Autodesk Inventor part; units mm, degrees
ref_plane "YZ Plane" through (0, 0, 0) normal (1, 0, 0) x (0, 1, 0)
ref_plane "XZ Plane" through (0, 0, 0) normal (0, 1, 0) x (-1, 0, 0)
ref_plane "XY Plane" through (0, 0, 0) normal (0, 0, 1) x (1, 0, 0)
sketch "Skizze1" plane through (0, 0, 0) normal (0, 0, 1) x (1, 0, 0)
  line L0 (-70, 25) -> (-70, 40)
  line L1 (-70, 40) -> (-80, 40)
  line L2 (-80, 40) -> (-80, 0)
  line L3 (-80, 0) -> (77, 0)
  line L4 (77, 0) -> (77, 25)
  line L5 (72, 25) -> (72, 23)
  line L6 (72, 23) -> (70, 23)
  line L7 (70, 23) -> (70, 25)
  line L8 (77, 25) -> (72, 25)
  line L9 (70, 25) -> (-70, 25)
  dimension "d0" = 80
  dimension "d1" = 10
  dimension "d2" = 50
  dimension "d3" = 46
  dimension "d7" = 2
  dimension "d8" = 5
  dimension "d13" = 140
revolve "Drehung1" add sketch "Skizze1" angle 360 about axis through (-80, 0, 0) along (1, 0, 0)
chamfer "Fase1" distance 2 angle 45 1 edges at (-80, -40, 0)
chamfer "Fase2" distance 2 angle 45 1 edges at (77, -25, 0)
properties part number "Boltx50"
Here's how the part is built. I have some questions about the finished solid (model axes, mm). A direction names the side the tool comes from. Give positions to 0.01 mm unless a question says otherwise; leave off trailing zeros. Order: outer loops, then holes, each group sorted by start corner. A loop starts at its lowest first (then second) coordinate and runs counter-clockwise, first axis right, second up. Notation, with made-up numbers: M -13.5,-6 L 7.5,-6 A17 ccw 7.5,0 Z; hole C -15.75,4.25 d3. An arc over 180 degrees is marked long. Answer as a JSON object with one key per item and string values. Group by question number.
1) I'm going to push flat-ended pins straight in: pin 1 Ø6 at (x, y) = (-52, -14.5) entering from +Z; pin 2 Ø2 at (x, y) = (-3, -5.5) entering from -Z; pin 3 Ø8 at (x, y) = (-42, -3.5) entering from +Z. Where does each tip first touch, or does it pass through?
2) On a 3-axis mill with a long thin cutter (end or side, diameter ignored), from which of +Z, -Z, +X, -X, +Y, -Y can I reach the whole of each face in a straight line? I mean faces 1 (the flat face through (-70, 17.22, 18.34)), 2 (the flat face through (77, 0, 0)), 3 (the flat face through (70, 22.1, -7.3)). Say none if no direction works.
3) We'd pull the mould along X, two halves only. Please class faces 4 (the flat face through (72, 22.1, -7.3)), 5 (the conical face through (-79.875, -4.963, 37.801)), 6 (the cylindrical face through (-74.06, -8.67, 39.05)): pulls with the +X half, pulls with the -X half, needs draft (parallel to the pull), parting line crosses it, or undercut.
4) Suppose I cut it at C-C, the plane x = 38. Write out the boundary of the cut face in (y, z), plus the area to 3 significant figures.
5) Please list where these lines run through material, in increasing order: L1, parallel to X at y = -24.5, z = -29; L2, parallel to Y at x = 21, z = -4.5; L3, parallel to Y at x = -34, z = -6. Write a range as [from, to].
6) Suppose I cut it at A-A, the plane y = 0. Write out the boundary of the cut face in (x, z).
Results found:
{
 "1": {"pin 1": "z = 22.2", "pin 2": "z = -24.59", "pin 3": "z = 25"},
 "2": {"face 1": "+X", "face 2": "+Z, -Z, +X, +Y, -Y", "face 3": "none"},
 "3": {"face 4": "undercut", "face 5": "pulls with the -X half", "face 6": "needs draft"},
 "4": {"outline": "C 0,0 d50", "area": "1,960 mm²"},
 "5": {"L1": "[-80, -70]", "L2": "[-24.59, 24.59]", "L3": "[-24.27, 24.27]"},
 "6": {"outline": "M -80,-38 L -78,-40 L -70,-40 L -70,-25 L 70,-25 L 70,-23 L 72,-23 L 72,-25 L 75,-25 L 77,-23 L 77,23 L 75,25 L 72,25 L 72,23 L 70,23 L 70,25 L -70,25 L -70,40 L -78,40 L -80,38 Z"}
}
